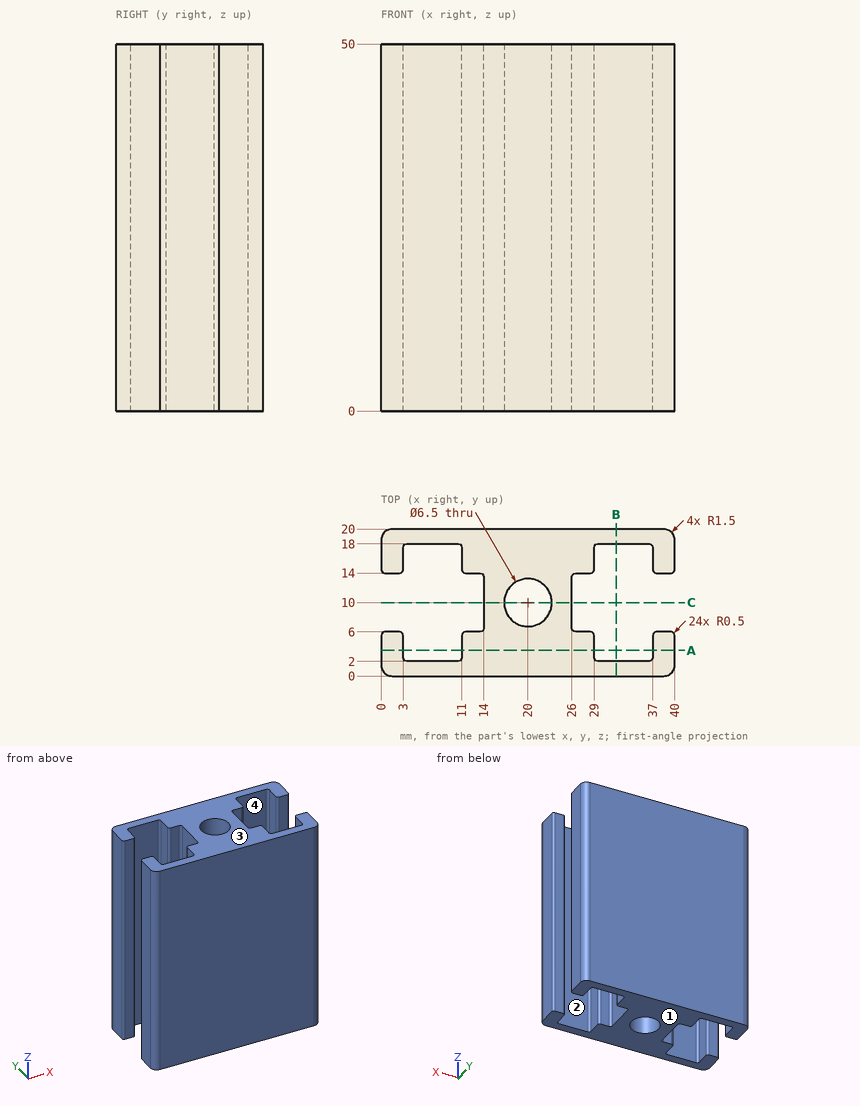
Answer from the drawing. Dimensions are ordinates in mm from the lowest x, y and z of the part. A direction names the side the tool comes from. Round coordinates to 2 decimals unless told otherwise and drop trailing zeros. Loops run counter-clockwise (first coordinate to the right, second up) from the corner with the lowest first, then second, coordinate; pieces in that order, holes last.
(1) The part is cut by section B-B, the plane x = 32. Give the vertices of the cut face in (y, z), and give its area (3 significant figures).
Computed values:
outline: (0, 0) - (2, 0) - (2, 50) - (0, 50) - close; (18, 0) - (20, 0) - (20, 50) - (18, 50) - close
area: 200 mm2
(2) The mould has two halves that part along X. Classify the marked faces 1 and 2: pulls with the +X half, pulls with the -X half, needs draft (parallel to the pull), parting line crosses it, or undercut.
Computed values:
face 1: needs draft
face 2: undercut
(3) For the marked faces 3 and 4, determine the directions among +Z, -Z, +X, -X, +Y, -Y from which every point of the face is accessible in a straight line to the end or side of a thin tool.
Computed values:
face 3: +Z, +X, -X, +Y, -Y
face 4: +Z, -Z
(4) Each of these flat-tipped pins is pushed along its axis until it touches: P1, Ø2, axis at y = 9, z = 28, coming from the +X side; P2, Ø2, axis at y = 9.5, z = 33.5, coming from the -X side. Where does it stop, or does it pass through?
Computed values:
P1: stops at x = 26
P2: stops at x = 14
(5) The part is cut by section C-C, the plane y = 10. Give the vertices of the cut face in (x, z).
Computed values:
outline: (14, 0) - (16.75, 0) - (16.75, 50) - (14, 50) - close; (23.25, 0) - (26, 0) - (26, 50) - (23.25, 50) - close
(6) The part is cut by section A-A, the plane y = 3.5. Give the vertices of the cut face in (x, z).
Computed values:
outline: (0, 0) - (3, 0) - (3, 50) - (0, 50) - close; (11, 0) - (29, 0) - (29, 50) - (11, 50) - close; (37, 0) - (40, 0) - (40, 50) - (37, 50) - close
(7) Find the intervals of material crossed by L1, parallel to X at y = 4, z = 37.5; L2, parallel to X at y = 10.25, z = 8; L3, parallel to Y at x = 34, z = 14, in increasing order.
Computed values:
L1: x = 0 to 3, 11 to 29, 37 to 40
L2: x = 14 to 16.76, 23.24 to 26
L3: y = 0 to 2, 18 to 20
